Autodesk Inventor part; units mm, degrees
ref_plane "YZ Plane" through (0, 0, 0) normal (1, 0, 0) x (0, 1, 0)
ref_plane "XZ Plane" through (0, 0, 0) normal (0, 1, 0) x (-1, 0, 0)
ref_plane "XY Plane" through (0, 0, 0) normal (0, 0, 1) x (1, 0, 0)
sketch "草图1" plane through (0, 0, 0) normal (0, 1, 0) x (-1, 0, 0)
  line L0 (77, 77) -> (-77, 77)
  line L1 (-77, 77) -> (-77, -77)
  line L2 (-77, -77) -> (77, -77)
  line L3 (77, -77) -> (77, 77)
  line L4 (0, 0) -> (0, -24)
  line L5 (0, 0) -> (17, 0)
  line L6 (75, 75) -> (-75, 75)
  line L7 (-75, 75) -> (-75, -75)
  line L8 (-75, -75) -> (75, -75)
  line L9 (75, -75) -> (75, 75)
  line L10 (-27, 6) -> (27, 6)
  line L11 (29, 4) -> (-29, 4)
  line L12 (29, 4) -> (29, 75)
  line L13 (-29, 4) -> (-29, 75)
  line L14 (27, 6) -> (27, 75)
  line L15 (-27, 6) -> (-27, 75)
  dimension "d1" = 154
  dimension "d2" = 154
  dimension "d3" = 150
  dimension "d4" = 150
  dimension "d5" = 54
  dimension "d6" = 58
  dimension "d7" = 71
  dimension "d8" = 69
sketch "草图4" plane through (0, 0, 0) normal (0, 1, 0) x (-1, 0, 0)
  line L0 (77, 77) -> (-77, 77)
  line L1 (-77, 77) -> (-77, -77)
  line L2 (-77, -77) -> (77, -77)
  line L3 (77, -77) -> (77, 77)
  line L4 (0, 0) -> (0, -178.4057)
  line L5 (0, 0) -> (-63.1988, 0)
  line L6 (75, 75) -> (-75, 75)
  line L7 (-75, 75) -> (-75, -75)
  line L8 (-75, -75) -> (75, -75)
  line L9 (75, -75) -> (75, 75)
  line L10 (-27, 6) -> (27, 6)
  line L11 (29, 4) -> (-29, 4)
  line L12 (29, 4) -> (29, 75)
  line L13 (-29, 4) -> (-29, 75)
  line L14 (27, 6) -> (27, 75)
  line L15 (-27, 6) -> (-27, 75)
  dimension "d11" = 154
  dimension "d12" = 154
  dimension "d13" = 150
  dimension "d14" = 150
  dimension "d15" = 54
  dimension "d16" = 58
  dimension "d17" = 71
  dimension "d18" = 69
sketch "草图5" plane through (0, 0, 0) normal (0, 1, 0) x (-1, 0, 0)
  line L0 (77, 77) -> (-77, 77)
  line L1 (-77, 77) -> (-77, -77)
  line L2 (-77, -77) -> (77, -77)
  line L3 (77, -77) -> (77, 77)
  line L4 (0, 0) -> (0, -24)
  line L5 (0, 0) -> (17, 0)
  line L6 (75, 75) -> (-75, 75)
  line L7 (-75, 75) -> (-75, -75)
  line L8 (-75, -75) -> (75, -75)
  line L9 (75, -75) -> (75, 75)
  line L10 (-27, 6) -> (27, 6)
  line L11 (29, 4) -> (-29, 4)
  line L12 (29, 4) -> (29, 75)
  line L13 (-29, 4) -> (-29, 75)
  line L14 (27, 6) -> (27, 75)
  line L15 (-27, 6) -> (-27, 75)
  dimension "d19" = 154
  dimension "d20" = 154
  dimension "d21" = 150
  dimension "d22" = 150
  dimension "d23" = 54
  dimension "d24" = 58
  dimension "d25" = 71
  dimension "d26" = 69
sketch "草图6" plane through (0, 0, 0) normal (0, 1, 0) x (-1, 0, 0)
  line L0 (0, 0) -> (0, -24)
  line L1 (0, 0) -> (17, 0)
  line L2 (-75, 75) -> (-75, -75)
  line L3 (-77, 77) -> (-77, -77)
  line L4 (29, 4) -> (-29, 4)
  line L5 (-27, 6) -> (27, 6)
  line L6 (75, 75) -> (-75, 75)
  line L7 (77, 77) -> (-77, 77)
  line L8 (29, 4) -> (29, 75)
  line L9 (27, 6) -> (27, 75)
  line L10 (-29, 4) -> (-29, 75)
  line L11 (-27, 6) -> (-27, 75)
  line L12 (-77, -77) -> (77, -77)
  line L13 (-75, -75) -> (75, -75)
  line L14 (77, -77) -> (77, 77)
  line L15 (75, -75) -> (75, 75)
  dimension "d27" = 154
  dimension "d28" = 154
  dimension "d29" = 150
  dimension "d30" = 150
  dimension "d31" = 54
  dimension "d32" = 58
  dimension "d33" = 71
  dimension "d34" = 69
extrude "拉伸2" add sketch "草图4" along normal blind 5 contours L3 L2 L1 L0 | L6 L15 L10 L14 L12 L11 L13
extrude "拉伸3" add sketch "草图1" against normal blind 10 contours L3 L2 L1 L0 | L9 L8 L7 L6 L13 L11 L12 | L12 L11 L13 L6 L15 L10 L14 | L14 L10 L15 L6
extrude "拉伸4" add sketch "草图5" along normal blind 50
sketch "草图7" plane through (-77, -10, 77) normal (0, 0, 1) x (1, 0, 0)
  line L0 (77, 10) -> (104, 10)
  line L1 (2, 10) -> (152, 10)
  line L2 (104, 10) -> (104, 25)
  line L3 (104, 25) -> (50, 25)
  line L4 (50, 25) -> (50, 10)
  line L5 (50, 10) -> (104, 10)
  line L6 (77, 10) -> (77, 15)
  line L7 (77, 15) -> (50, 15)
  line L8 (60, 15) -> (60, 25)
  line L9 (60, 25) -> (50, 25)
  line L10 (60, 25) -> (50, 25)
  line L11 (60, 25) -> (71.5, 25)
  line L12 (71.5, 25) -> (71.5, 15)
  line L13 (50, 25) -> (91, 25)
  line L14 (50, 25) -> (100, 25)
  line L15 (91, 25) -> (91, 15)
  line L16 (91, 15) -> (100, 15)
  line L17 (100, 15) -> (100, 25)
  dimension "d42" = 15
  dimension "d43" = 54
  dimension "d44" = 5
  dimension "d45" = 10
  dimension "d46" = 10
  dimension "d47" = 11.5
  dimension "d48" = 41
  dimension "d49" = 50
  dimension "d50" = 10
extrude "拉伸5" cut sketch "草图7" against normal blind 3 contours L7 L8 L3 L12 | L17 L16 L15 L3
sketch "草图8" plane through (77, -10, -77) normal (0, 0, -1) x (-1, 0, 0)
  line L0 (77, 10) -> (112.5, 10)
  line L1 (50, 10) -> (104, 10)
  line L2 (112.5, 10) -> (112.5, 37)
  line L3 (112.5, 37) -> (41.5, 37)
  line L4 (41.5, 37) -> (41.5, 10)
  line L5 (41.5, 10) -> (77, 10)
  dimension "d53" = 35.5
  dimension "d54" = 27
  dimension "d55" = 71
extrude "拉伸6" cut sketch "草图8" against normal blind 3
sketch "草图9" plane through (0, 0, 0) normal (0, 1, 0) x (1, 0, 0)
  line L0 (0, 0) -> (0, 10)
  line L1 (0, 10) -> (-18, 10)
  line L2 (0, 10) -> (8, 10)
  line L3 (8, 10) -> (8, 12)
  line L4 (8, 12) -> (-18, 12)
  line L5 (-18, 12) -> (-18, 10)
  line L6 (0, 12) -> (0, 27.6)
  line L7 (0, 27.6) -> (-18, 27.6)
  line L8 (-18, 27.6) -> (-18, 29.6)
  line L9 (-18, 29.6) -> (8, 29.6)
  line L10 (8, 29.6) -> (8, 27.6)
  line L11 (8, 27.6) -> (0, 27.6)
  line L12 (-18, 27.6) -> (-18, 12)
  line L13 (-18, 12) -> (-13, 12)
  line L14 (-13, 12) -> (-13, 27.6)
  line L15 (-18, 27.6) -> (-13, 27.6)
  dimension "d58" = 10
  dimension "d59" = 18
  dimension "d60" = 8
  dimension "d61" = 15.6
  dimension "d62" = 2
  dimension "d75" = 5
extrude "拉伸8" add sketch "草图9" along normal blind 15 contours L1 L5 L4 L3 L2 | L12 L7 L14 L4 | L8 L9 L10 L11 L7
sketch "草图14" plane through (0, 15, 0) normal (0, 1, 0) x (1, 0, 0)
  line L0 (-13, 12) -> (-13, 27.6)
  line L1 (-13, 27.6) -> (-13, 12)
  line L2 (-13, 12) -> (-18, 12)
  line L3 (-18, 12) -> (-18, 27.6)
  line L4 (-18, 27.6) -> (-13, 27.6)
  point P0 (0, 0)
extrude "拉伸9" cut sketch "草图14" against normal blind 2
sketch "草图15" plane through (0, 13, 0) normal (0, 1, 0) x (1, 0, 0)
  line L0 (-18, 27.6) -> (8, 27.6)
  line L1 (-18, 27.6) -> (-15.5, 27.6)
  line L2 (-15.5, 27.6) -> (-15.5, 23.8)
  line L3 (-15.5, 23.8) -> (-15.5, 15.8)
  circle A0 centre (-15.5, 23.8) radius 1.5
  circle A1 centre (-15.5, 15.8) radius 1.5
  point P0 (0, 0)
  dimension "d80" = 2.5
  dimension "d81" = 3.8
  dimension "d82" = 8
  dimension "d83" = 3
  dimension "d84" = 3
extrude "拉伸10" cut sketch "草图15" against normal blind 13
properties part number "底座"
The model under review builds one solid part; all positions refer to its coordinate system, in mm. A direction names the side the tool comes from. Round coordinates to 2 decimals unless told otherwise and drop trailing zeros. Loops run counter-clockwise (first coordinate to the right, second up) from the corner with the lowest first, then second, coordinate; pieces in that order, holes last.
Item 1: Take a section at D-D (z = 22). Write out the cut boundary in (x, y), then the cut area to 3 significant figures.
Determined:
outline: (-77, -10) - (77, -10) - (77, 50) - (75, 50) - (75, 0) - (29, 0) - (29, 5) - (27, 5) - (27, 0) - (-27, 0) - (-27, 5) - (-29, 5) - (-29, 0) - (-75, 0) - (-75, 50) - (-77, 50) - close
area: 1,760 mm2
Item 2: Take a section at C-C (x = 48.5). Write out the cut boundary in (y, z), then the cut area to 3 significant figures.
Determined:
outline: (-10, -77) - (50, -77) - (50, -75) - (0, -75) - (0, 75) - (50, 75) - (50, 77) - (-10, 77) - close
area: 1,740 mm2
Item 3: Clearance check with flat-ended pins moving along their axes: pin 1 Ø1.5 at (x, y) = (-11.5, 3) entering from -Z; pin 2 Ø5 at (x, z) = (25.5, 7.5) entering from +Y; pin 3 Ø2 at (x, z) = (-34.5, 8.5) entering from +Y. State where each tip first meets the part, or that it passes through.
Determined:
pin 1: stops at z = -29.6
pin 2: stops at y = 5
pin 3: stops at y = 0
Item 4: Mouldability with a two-part tool opening along Z and no side actions: class faces 4 (the face through (1, 33, -77)), 5 (the face through (1, -10, 1)), 6 (the face through (-27, 2, 40)), 7 (the face through (-75, 25, -1)) as released by +Z, released by -Z, zero draft, split by the parting line, or undercut.
Determined:
face 4: released by -Z
face 5: zero draft
face 6: undercut
face 7: undercut
Item 5: For faces 1 (the face through (-13, 6, -20)), 2 (the face through (29, 2, 39)), 3 (the face through (-1, 20, 77)), list the 3-axis set-ups (+Z, -Z, +X, -X, +Y, -Y) from which the entire face can be reached by the end or side of a thin tool; tool diameter is ignored.
Determined:
face 1: +Y
face 2: -Z, +Y
face 3: +Z, +X, -X, +Y, -Y
Item 6: For line 1 (X direction, y = 10.5, z = -15.8); line 2 (Z direction, x = -15.5, y = 7.75); line 3 (Z direction, x = -15.5, y = 3.25), list the stretches that pass through material, from the lowest coordinate up.
Determined:
line 1: x = -77 to -75, -18 to -17, -14 to -13, 75 to 77
line 2: z = -29.6 to -25.3, -22.3 to -17.3, -14.3 to -10
line 3: z = -29.6 to -25.3, -22.3 to -17.3, -14.3 to -10, 4 to 6, 75 to 77
Item 7: Take a section at A-A (y = 3). Give the number of separate pieces and of enclosed holes in the cut face, then the cut area to 3 significant figures.
Determined:
separate pieces: 2
enclosed holes: 3
area: 1,630 mm2
Item 8: Take a section at B-B (y = 44). Write out the cut boundary in (x, z), then the cut area to 3 significant figures.
Determined:
outline: (-77, -77) - (77, -77) - (77, 77) - (-77, 77) - close; hole (-75, -75) - (75, -75) - (75, 75) - (-75, 75) - close
area: 1,220 mm2
